Check sheet for the modelled part. Datum: model origin and axes. Units: mm. A direction names the side the tool comes from. Give positions to 0.01 mm unless a question says otherwise; leave off trailing zeros. Loops run counter-clockwise (first coordinate to the right, second up) from the corner with the lowest first, then second, coordinate; pieces in that order, holes last. Notation, with made-up numbers: (89, 47.5) -> (111, 47.5) arc R26 ccw to (111, 70.5) -> close; hole circle Ø4 at (3.25, 40.25). An arc over 180 degrees is marked (long way). Answer as CSV lines item,"result". Start each with the question number.
(1) Access from +Z, -Z, +X, -X, +Y, -Y to the whole of each face (thin tool, end or side, straight path). Record for faces 4 (the face through (-7.3, 1, -5.6)), 5 (the face through (-7, 0, -7)).
(2) Gauge pin test, flat ends, axial feed: pin 1 Ø5 at (y, z) = (6, 10) entering from -X; pin 2 Ø8 at (x, z) = (0.5, -3) entering from -Y; pin 3 Ø4 at (x, z) = (6, -5.5) entering from +Y; pin 4 Ø12 at (x, z) = (9, -6) entering from -Y. Record the tip position at first contact, or that the pin passes through.
(3) Material ranges on line 1 (Z direction, x = 0, y = 0.7); line 2 (Z direction, x = 0, y = 1); line 3 (Y direction, x = -7.5, z = -0.25), recorded low to high. Write a range as from..to.
(4) Section check B-B on y = 9.25. Enter the section's corners in (x, z), plus the area to 3 significant figures.
(5) Release check for a two-part mould opening along X. For faces 1 (the face through (11.95, 2.74, 4.95)), 2 (the face through (0, 8, 0)), 3 (the face through (0, 2, 0)) record: pulls with the +X half, pulls with the -X half, needs draft (parallel to the pull), parting line crosses it, or undercut.
(6) Section check C-C on y = 1.25. Enter the section's corners in (x, z).
(7) Section check D-D on y = 3.75. Enter the section's corners in (x, z).
(8) Section check A-A on x = 0. Enter the section's corners in (y, z), plus the area to 3 significant figures.
from build123d import *

# Parameters (mm, degrees)
SKETCH1_R               = 12.5
BOSS_EXTRUDE1_DEPTH     = 10
BOSS_EXTRUDE1_TAPER     = -9
SKETCH2_R               = 9.2
CUT_EXTRUDE1_DEPTH      = 2
SKETCH3_R               = 61.5
CUT_EXTRUDE2_DEPTH      = 15.083844503
CUT_EXTRUDE2_DEPTH_BACK = 15.083844503


with BuildPart() as part:
    # Sketch1 → Boss-Extrude1 (new body)
    with BuildSketch(Plane(origin=(0, 0, 0), x_dir=(1, 0, 0), z_dir=(0, 1, 0))):
        Circle(SKETCH1_R)
    extrude(amount=BOSS_EXTRUDE1_DEPTH, taper=BOSS_EXTRUDE1_TAPER)

    # Sketch2 → Cut-Extrude1 (cut)
    with BuildSketch(Plane.XZ):
        Circle(SKETCH2_R)
    extrude(amount=-CUT_EXTRUDE1_DEPTH, mode=Mode.SUBTRACT)

    # Sketch3 → Cut-Extrude2 (cut, two sides)
    with BuildSketch(Plane(origin=(0, 0, 0), x_dir=(0, 0, -1), z_dir=(1, 0, 0))) as cut_extrude2_sk:
        with Locations((0, 69.5)):
            Circle(SKETCH3_R)
    extrude(amount=CUT_EXTRUDE2_DEPTH, mode=Mode.SUBTRACT)
    extrude(cut_extrude2_sk.sketch, amount=-CUT_EXTRUDE2_DEPTH_BACK, mode=Mode.SUBTRACT)


solid = part.part
Working result:
1,face 4,"-Y"
1,face 5,"+Z, -Z, +X, -X, -Y"
2,pin 1,"stops at x = -11.23"
2,pin 2,"stops at y = 2"
2,pin 3,"stops at y = 8.46"
2,pin 4,"stops at y = 0"
3,line 1,"z = -12.61..-9.2, 9.2..12.61"
3,line 2,"z = -12.66..-9.2, 9.2..12.66"
3,line 3,"y = 2..8"
4,outline,"(-6.54, -12.34) arc R13.97 ccw to (6.54, -12.34) -> close; (-6.54, 12.34) -> (6.54, 12.34) arc R13.97 ccw to start"
4,area,"28.8 mm^2"
5,face 1,"parting line crosses it"
5,face 2,"needs draft"
5,face 3,"undercut"
6,outline,"circle Ø25.4 at (0, 0); hole circle Ø18.4 at (0, 0)"
7,outline,"circle Ø26.19 at (0, 0)"
8,outline,"(0, -12.5) -> (9.62, -14.02) arc R61.5 cw to (9.62, 14.02) -> (0, 12.5) -> (0, 9.2) -> (2, 9.2) -> (2, -9.2) -> (0, -9.2) -> close"
8,area,"188 mm^2"
